Check sheet for the drawn part. Datum: minimum x, y, z corner. Units: mm. Round coordinates to 2 decimals unless told otherwise and drop trailing zeros. Write each loop counter-clockwise with the first axis right and the second up, starting at its lowest first coordinate (ties: lowest second). Pieces come first, ordered by that corner, then holes. Notation, with made-up numbers: M 12,45 L 35,45 A23 ccw 35,81 Z; hole C 70.25,30 d10. An arc over 180 degrees is marked long. One line per item, written item: value. Start each with the question number.
Item 1: Section check C-C, the plane x = 71. Record the cut outline in (y, z).
Item 2: Thickness scan on probe 1 along X at (y, z) = (5, 25); probe 2 along X at (y, z) = (1.4, 15.75); probe 3 along X at (y, z) = (2.2, 34.25). Record the ranges inside material, lowest first. Write a range as from..to.
Item 3: Section check B-B, the plane z = 15.75. Record the cut outline in (x, y), then the cut area to 3 significant figures.
Item 4: Section check D-D, the plane z = 31.5. Record the cut outline in (x, y).
Item 5: Gauge pin test, flat ends, axial feed: pin 1 (2.5 mm diameter, centred on x = 8, z = 25, fed in from -Y); pin 2 (25 mm diameter, centred on x = 30, z = 25.5, fed in from +Y). Record the tip position at first contact, or that the pin passes through.
Item 6: Section check A-A, the plane x = 8. Record the cut outline in (y, z).
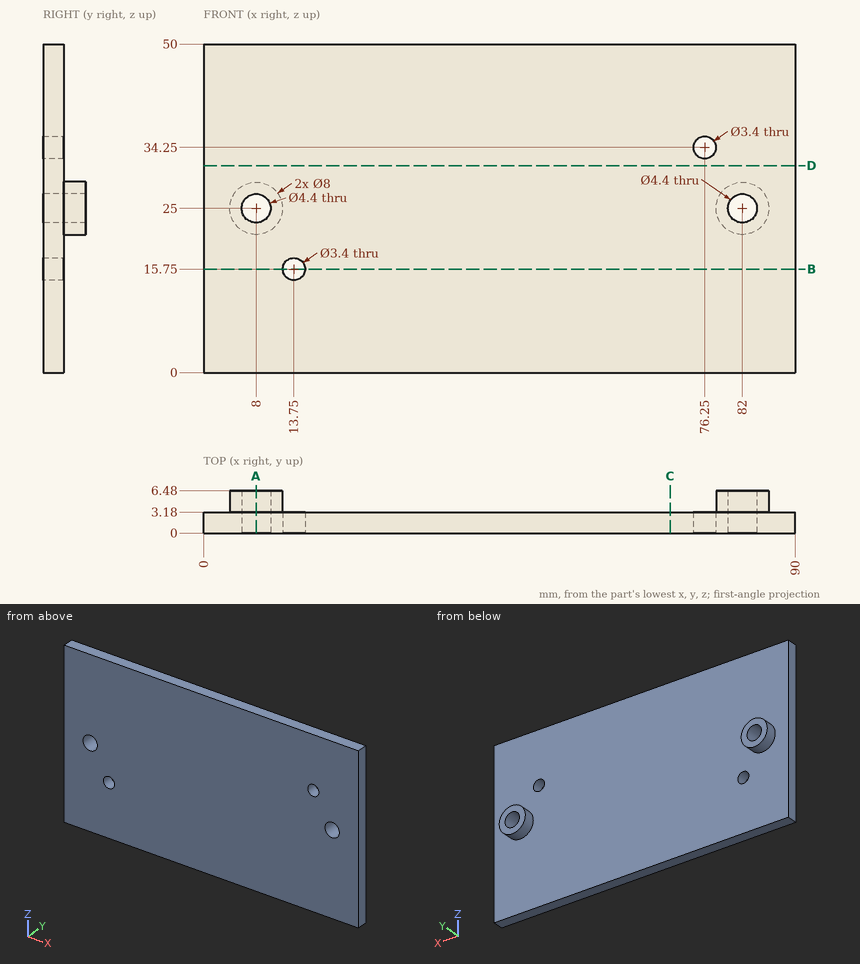
Response values:
1. outline: M 0,0 L 3.18,0 L 3.18,50 L 0,50 Z
2. probe 1: x = 4..5.8, 10.2..12, 78..79.8, 84.2..86
2. probe 2: x = 0..12.05, 15.45..90
2. probe 3: x = 0..74.55, 77.95..90
3. outline: M 0,0 L 12.05,0 L 12.05,3.18 L 0,3.18 Z; M 15.45,0 L 90,0 L 90,3.18 L 15.45,3.18 Z
3. area: 275 mm2
4. outline: M 0,0 L 90,0 L 90,3.18 L 0,3.18 Z
5. pin 1: passes through
5. pin 2: stops at y = 3.18
6. outline: M 0,0 L 3.18,0 L 3.18,21 L 6.48,21 L 6.48,22.8 L 0,22.8 Z; M 0,27.2 L 6.48,27.2 L 6.48,29 L 3.18,29 L 3.18,50 L 0,50 Z
